```python
from build123d import *

# Parameters (mm, degrees)
F2_R    = 5.08
F3_SIZE = 5.08


with BuildPart() as f1:
    # F0 (on Right) → F1 (revolve)
    with BuildSketch(Plane.YZ):
        Polygon((-57.615455, 0), (46.00529, 0), (36.136646, 21.914188), (15.238347, 21.914188), (6.530722, 10.594275), (-29.170545, 10.594275), (-37.587918, 30.331559), (-57.615455, 30.331559), align=None)
    revolve(axis=Axis((0, 3.918434, 0), (0, -1, 0)))

    # F2
    f2_edges = [f1.edges().sort_by_distance(p)[0] for p in [
        (0, 36.136646, -21.914188),
        (0, 15.238347, -21.914188),
    ]]
    fillet(f2_edges, radius=F2_R)

    # F3
    f3_edges = [f1.edges().sort_by_distance(p)[0] for p in [
        (0, -37.587918, -30.331559),
    ]]
    chamfer(f3_edges, length=F3_SIZE)


solid = f1.part
```
For this review, take the finished solid that the model builds, in its own axes (mm). A direction names the side the tool comes from. Coordinates: 2 decimals unless noted, no trailing zeros. Write each loop counter-clockwise with the first axis right and the second up, starting at its lowest first coordinate (ties: lowest second). Pieces come first, ordered by that corner, then holes.
(1) Add section A-A on y = -4.5. Give the boundary of the cut face in (x, z), then the cut area to 3 significant figures.
(2) Wall thickness on probe 1 along Y at (x, z) = (-6, -14); probe 2 along Y at (x, z) = (14.5, 3.5); probe 3 along Y at (x, z) = (24, 9.5): over which ranges is each line inside the solid? List them lowest first.
(3) Add section B-B on y = 30.5. Give the boundary of the cut face in (x, z).
(4) For pin 1 Ø3 at (x, z) = (16.5, 2.5) entering from +Y; pin 2 Ø3 at (y, z) = (-22.5, 2.5) entering from +X; pin 3 Ø12 at (x, z) = (18, -10) entering from +Y, all flat-tipped, find the tip position at first contact; note any pin that passes through.
(5) Tool access review of faces 4 (the face through (8.393, 25.191, 20.243)), 5 (the face through (-3.47, -29.57, 11)), 6 (the face through (11.617, -50.246, 28.019)): name each direction out of +Z, -Z, +X, -X, +Y, -Y from which nothing blocks a thin tool from reaching the whole face with its end or side.
(6) The part is to be moulded in two halves that separate along Y. For faces 1 (the face through (-7.16, -11.57, -7.81)), 2 (the face through (0, -57.615, 0)), 3 (the face through (0.453, 45.472, 1.093)), say which applies: +Y half, -Y half, draft (parallel to the pull), parting line (faces both ways), or undercut.
Answer sheet:
1. outline: circle Ø21.19 at (0, 0)
1. area: 353 mm2
2. probe 1: y = -57.62 to -31.15, 10.1 to 39.15
2. probe 2: y = -57.62 to -31.01, 9.86 to 39.29
2. probe 3: y = -57.62 to -35.83
3. outline: circle Ø43.83 at (0, 0)
4. pin 1: stops at y = 39.17
4. pin 2: stops at x = 10.55
4. pin 3: stops at y = 39.43
5. face 4: +Y
5. face 5: none
5. face 6: +Y, -Y
6. face 1: undercut
6. face 2: -Y half
6. face 3: +Y half
